```python
from build123d import *

# Parameters (mm, degrees)
F0_W     = 25.4
F0_H     = 12.7
F1_DEPTH = 12.7
F3_D     = 5.1054
F5_DEPTH = 25.4
F7_DEPTH = 25.4
F9_DEPTH = 25.4


with BuildPart() as f1:
    # F0 (on Top) → F1 (new body)
    with BuildSketch(Plane.XY):
        with Locations((0.563834, -1.404666)):
            Rectangle(F0_W, F0_H)
    extrude(amount=F1_DEPTH)

    # F3 (through all)
    with Locations(Plane(origin=(0, 0, 0), x_dir=(1, 0, 0), z_dir=(0, 0, -1))):
        with Locations((0.563834, 0)):
            Hole(F3_D / 2)

    # F4 (on face) → F5 (cut)
    with BuildSketch(Plane.XY.offset(12.7)):
        Polygon((-9.596166, -2.537197), (-9.596166, -5.214666), (10.723834, -5.214666), (10.723834, -2.854676), (8.765497, -2.854676), (8.765497, -4.253724), (-7.137803, -4.253724), (-7.137803, -2.854676), align=None)
    extrude(amount=-F5_DEPTH, mode=Mode.SUBTRACT)

    # F6 (on face) → F7 (cut)
    with BuildSketch(Plane.XY.offset(12.7)):
        Polygon((-9.650016, 2.781621), (-9.650016, 0), (-6.187561, 0), (-3.966114, -1.597365), (-3.966114, 0), (-5.780214, 2.781621), (-8.122463, 1.254068), (-8.122463, 2.781621), align=None)
    extrude(amount=-F7_DEPTH, mode=Mode.SUBTRACT)

    # F8 (on face) → F9 (cut)
    with BuildSketch(Plane.XY.offset(12.7)):
        Polygon((9.393484, 1.865089), (6.847562, 1.865089), (7.967768, 1.050394), (8.986138, 0), (7.764094, 0), (4.810824, 1.050394), (6.643889, -1.088181), (10.819201, -1.088181), align=None)
    extrude(amount=-F9_DEPTH, mode=Mode.SUBTRACT)


solid = f1.part
```
The model under review builds one solid part; all positions refer to its coordinate system, in mm. A direction names the side the tool comes from. Round coordinates to 2 decimals unless told otherwise and drop trailing zeros. Write each loop counter-clockwise with the first axis right and the second up, starting at its lowest first coordinate (ties: lowest second). Pieces come first, ordered by that corner, then holes.
(1) Insertion check: pin 1 (6 mm diameter, centred on x = -1, y = -4.5, fed in from +Z). The pin has a flat end and moves straight along its axis. Give the tip position at first contact, or say it passes through.
(2) We need section B-B on z = 2. Give the number of separate pieces and of enclosed holes in the cut face, and give its area (3 significant figures).
(3) We need section C-C on x = 2. Give the boundary of the cut face in (y, z), and give its area (3 significant figures).
(4) We need section D-D on x = 5.75. Give the boundary of the cut face in (y, z).
(5) Mouldability with a two-part tool opening along X and no side actions: class faces 1 (the flat face through (13.264, -1, 6)), 2 (the flat face through (0, -7.755, 6)), 3 (the flat face through (-9, 2.782, 6)) as +X half, -X half, draft (parallel to the pull), parting line (faces both ways), or undercut.
(6) We need section A-A on y = 0.25. Give the boundary of the cut face in (x, z).
(7) Machinability: for faces 4 (the flat face through (0, -3, 0)), 5 (the flat face through (-9.596, -4, 6)), which of the approach directions +Z, -Z, +X, -X, +Y, -Y give a long, thin tool a straight path to every point of the face, cutting with its end or side? Answer none if there is none.
(8) Wall thickness on L1, parallel to Y at x = -9.25, z = 1.75; L2, parallel to Y at x = -5.25, z = 7.5; L3, parallel to X at y = -4.5, z = 8.5: over which ranges is each line inside the solid? List them lowest first.
Findings below:
1. pin 1: stops at z = 12.7
2. separate pieces: 1
2. enclosed holes: 4
2. area: 253 mm2
3. outline: (-7.75, 0) - (-5.21, 0) - (-5.21, 12.7) - (-7.75, 12.7) - close; (-4.25, 0) - (-2.11, 0) - (-2.11, 12.7) - (-4.25, 12.7) - close; (2.11, 0) - (4.95, 0) - (4.95, 12.7) - (2.11, 12.7) - close
3. area: 95.5 mm2
4. outline: (-7.75, 0) - (-5.21, 0) - (-5.21, 12.7) - (-7.75, 12.7) - close; (-4.25, 0) - (-0.05, 0) - (-0.05, 12.7) - (-4.25, 12.7) - close; (0.72, 0) - (4.95, 0) - (4.95, 12.7) - (0.72, 12.7) - close
5. face 1: +X half
5. face 2: draft
5. face 3: undercut
6. outline: (-12.14, 0) - (-9.65, 0) - (-9.65, 12.7) - (-12.14, 12.7) - close; (-4.13, 0) - (-1.98, 0) - (-1.98, 12.7) - (-4.13, 12.7) - close; (3.1, 0) - (5.5, 0) - (5.5, 12.7) - (3.1, 12.7) - close; (7.06, 0) - (8.74, 0) - (8.74, 12.7) - (7.06, 12.7) - close; (10.17, 0) - (13.26, 0) - (13.26, 12.7) - (10.17, 12.7) - close
7. face 4: -Z, +X, -X, +Y, -Y
7. face 5: +Z, -Z
8. L1: y = -7.75 to -5.21, -2.58 to 0, 2.78 to 4.95
8. L2: y = -7.75 to -5.21, -4.25 to -0.67, 1.97 to 4.95
8. L3: x = -12.14 to -9.6, 10.72 to 13.26
